Check sheet for the modelled part. Datum: model origin and axes. Units: mm. A direction names the side the tool comes from. Coordinates: 2 decimals unless noted, no trailing zeros. Order: outer loops, then holes, each group sorted by start corner. A loop starts at its lowest first (then second) coordinate and runs counter-clockwise, first axis right, second up.
1. Cross-section at B-B (y = 2.75). Enter the section's corners in (x, z).
2. Set-up check for faces 1 (the flat face through (0, 5, 3)), 2 (the cylindrical face through (2.958, 12.599, 9.815)), 3 (the flat face through (4.54, 10.05, 4.99)): record each of +Z, -Z, +X, -X, +Y, -Y from which the full face is reachable in a straight line by a thin tool's end or side.
3. Cross-section at A-A (z = 5.25). Enter the section's corners in (x, y) (3 decimals).
4. Thickness scan on line 1 (Y direction, x = 0, z = 5.5); line 2 (Y direction, x = 5.75, z = 8.75); line 3 (Z direction, x = -2.75, y = 14). Record the ranges inside material, lowest first.
5. Cross-section at D-D (z = 9.75). Enter the section's corners in (x, y).
6. Draft check along Y on faces 4 (the flat face through (-4.494, 10.114, 4.993)), 5 (the cylindrical face through (-2.271, 14.388, 9.815)), 6 (the flat face through (-5, 2.971, 5)). Enter one of: released by +Y, released by -Y, zero draft, split by the parting line, or undercut.
7. Gauge pin test, flat ends, axial feed: pin 1 Ø0.7 at (x, z) = (5, 3.5) entering from -Y; pin 2 Ø1 at (x, z) = (1.5, 1.5) entering from +Y; pin 3 Ø1.5 at (x, y) = (3.5, 3) entering from +Z. Record the tip position at first contact, or that the pin passes through.
8. Cross-section at C-C (z = 8.5). Enter the section's corners in (x, y).
```python
from build123d import *

# Parameters (mm, degrees)
F1_DEPTH = 10.1
F2_W     = 6.35
F2_H     = 1.778
F3_DEPTH = 4.318
F4_DEPTH = 7
F6_R     = 1


with BuildPart() as f1:
    # F0 (on Top) → F1 (new body)
    with BuildSketch(Plane.XY):
        Polygon((-2.708949, 0), (0, 0), (2.708949, 0), (2.708949, 2.971315), (7.713426, 2.971315), (4.857096, 7.86788), (6.097892, 7.86788), (2.933446, 12.298105), (4.174241, 12.298105), (0, 18), (-4.174241, 12.298105), (-2.933446, 12.298105), (-6.097892, 7.86788), (-4.857096, 7.86788), (-7.713426, 2.971315), (-2.708949, 2.971315), align=None)
    extrude(amount=F1_DEPTH)

    # F2 (on face) → F3 (cut)
    with BuildSketch(Plane(origin=(0, 0, 0), x_dir=(1, 0, 0), z_dir=(0, 0, -1))):
        with Locations((0, -5.889)):
            Rectangle(F2_W, F2_H)
    extrude(amount=-F3_DEPTH, mode=Mode.SUBTRACT)

    # F2 (on face) → F4 (cut)
    with BuildSketch(Plane(origin=(0, 0, 0), x_dir=(1, 0, 0), z_dir=(0, 0, -1))):
        with Locations((0, -5.889)):
            Rectangle(F2_W, F2_H)
    extrude(amount=-F4_DEPTH, mode=Mode.SUBTRACT)

    # F6
    f6_edges = [f1.edges().sort_by_distance(p)[0] for p in [
        (0, 18, 5.05),
        (-6.285261, 5.419597, 10.1),
        (-5.211187, 2.971315, 10.1),
        (-2.708949, 1.485657, 10.1),
        (0, 0, 10.1),
        (2.708949, 1.485657, 10.1),
        (5.211187, 2.971315, 10.1),
        (6.285261, 5.419597, 10.1),
        (5.477494, 7.86788, 10.1),
        (4.515669, 10.082993, 10.1),
        (3.553843, 12.298105, 10.1),
        (2.087121, 15.149053, 10.1),
        (-2.087121, 15.149053, 10.1),
        (-3.553843, 12.298105, 10.1),
        (-4.515669, 10.082993, 10.1),
        (-5.477494, 7.86788, 10.1),
        (4.515669, 10.082993, 0),
        (2.087121, 15.149053, 0),
        (-2.087121, 15.149053, 0),
        (-4.515669, 10.082993, 0),
        (-3.553843, 12.298105, 0),
        (-6.285261, 5.419597, 0),
        (-5.477494, 7.86788, 0),
        (-5.211187, 2.971315, 0),
        (-2.708949, 1.485657, 0),
        (0, 0, 0),
        (2.708949, 1.485657, 0),
        (5.211187, 2.971315, 0),
        (6.285261, 5.419597, 0),
    ]]
    fillet(f6_edges, radius=F6_R)


solid = f1.part
```
Data:
1. outline: (-2.71, 1) arc R1 ccw to (-1.71, 0) - (1.71, 0) arc R1 ccw to (2.71, 1) - (2.71, 9.1) arc R1 ccw to (1.71, 10.1) - (-1.71, 10.1) arc R1 ccw to (-2.71, 9.1) - close
2. face 1: -Z
2. face 2: +Z, +X
2. face 3: +Z, -Z, +X
3. outline: (-7.713, 2.971) - (-2.709, 2.971) - (-2.709, 0) - (2.709, 0) - (2.709, 2.971) - (7.713, 2.971) - (4.857, 7.868) - (6.098, 7.868) - (2.933, 12.298) - (4.174, 12.298) - (0.807, 16.898) arc R1 ccw to (-0.807, 16.898) - (-4.174, 12.298) - (-2.933, 12.298) - (-6.098, 7.868) - (-4.857, 7.868) - close; hole (-3.175, 5) - (3.175, 5) - (3.175, 6.778) - (-3.175, 6.778) - close
4. line 1: y = 0 to 5, 6.78 to 17.31
4. line 2: y = 2.97 to 6.34, 7.87 to 8.35
4. line 3: z = 0.48 to 9.62
5. outline: (-7.3, 3.21) - (-2.47, 3.21) - (-2.47, 0.24) - (2.47, 0.24) - (2.47, 3.21) - (7.3, 3.21) - (4.44, 8.11) - (5.63, 8.11) - (2.47, 12.54) - (3.7, 12.54) - (0.61, 16.76) arc R0.76 ccw to (-0.61, 16.76) - (-3.7, 12.54) - (-2.47, 12.54) - (-5.63, 8.11) - (-4.44, 8.11) - close
6. face 4: undercut
6. face 5: released by +Y
6. face 6: released by -Y
7. pin 1: stops at y = 2.97
7. pin 2: stops at y = 16.63
7. pin 3: stops at z = 10.08
8. outline: (-7.71, 2.97) - (-2.71, 2.97) - (-2.71, 0) - (2.71, 0) - (2.71, 2.97) - (7.71, 2.97) - (4.86, 7.87) - (6.1, 7.87) - (2.93, 12.3) - (4.17, 12.3) - (0.81, 16.9) arc R1 ccw to (-0.81, 16.9) - (-4.17, 12.3) - (-2.93, 12.3) - (-6.1, 7.87) - (-4.86, 7.87) - close
